Check sheet for the drawn part. Datum: minimum x, y, z corner. Units: mm. A direction names the side the tool comes from. Give positions to 0.01 mm unless a question says otherwise; leave off trailing zeros. Write each loop counter-clockwise with the first axis right and the second up, starting at its lowest first coordinate (ties: lowest second). Pieces come first, ordered by that corner, then holes. Notation, with made-up numbers: M 82,28.5 L 116,28.5 A18 ccw 116,34.5 Z; hole C -40,-39 d3. An arc over 180 degrees is marked long. Use CSV: the item, a comma, the result in double quotes. Start each with the question number.
1. Access from +Z, -Z, +X, -X, +Y, -Y to the whole of each face (thin tool, end or side, straight path). Record for the marked faces 1, 2 and 3.
2. Cross-section at B-B, the plane z = 13.7. Enter the section's corners in (x, y).
3. Depth check by flat-ended pin: P1, Ø5, axis at x = 3.5, z = 14, coming from the -Y side; P2, Ø12, axis at x = 6.5, y = 39, coming from the +Z side; P3, Ø12, axis at y = 25.5, z = 5, coming from the -X side. Enter the tip coordinate at first touch or a pass-through.
4. Cross-section at C-C, the plane y = 18. Enter the section's corners in (x, z), and give its area (3 significant figures).
5. Cross-section at A-A, the plane x = 13.7. Enter the section's corners in (y, z).
6. Cross-section at D-D, the plane y = 43.5. Enter the section's corners in (x, z).
7. Scan lines: line 1 (Y direction, x = 13, z = 20.75); line 2 (Y direction, x = 17.5, z = 12); line 3 (X direction, y = 6.5, z = 14.75). Record each from-to range of solid material in increasing order.
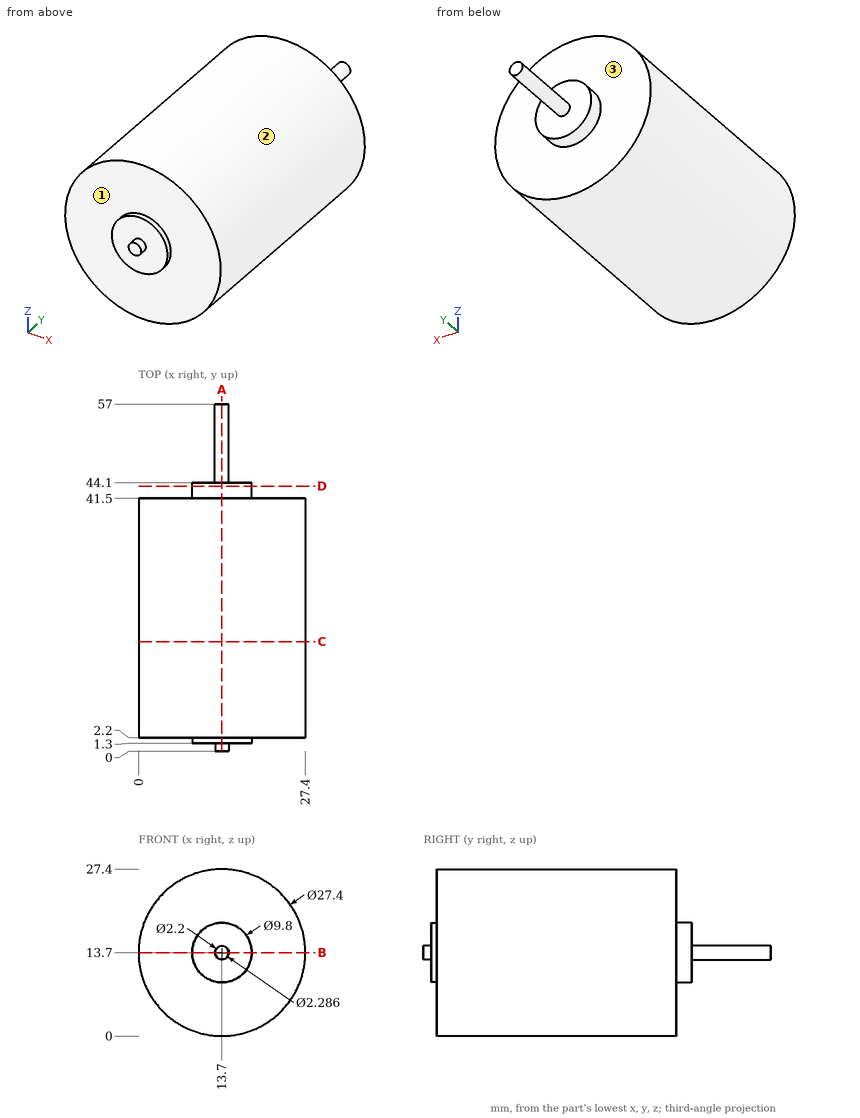
Worked answers:
1,face 1,"-Y"
1,face 2,"+Y, -Y"
1,face 3,"+Y"
2,outline,"M 0,2.2 L 8.8,2.2 L 8.8,1.3 L 12.6,1.3 L 12.6,0 L 14.8,0 L 14.8,1.3 L 18.6,1.3 L 18.6,2.2 L 27.4,2.2 L 27.4,41.5 L 18.6,41.5 L 18.6,44.1 L 14.84,44.1 L 14.84,57 L 12.56,57 L 12.56,44.1 L 8.8,44.1 L 8.8,41.5 L 0,41.5 Z"
3,P1,"stops at y = 2.2"
3,P2,"stops at z = 27.35"
3,P3,"stops at x = 0.27"
4,outline,"C 13.7,13.7 d27.4"
4,area,"590 mm^2"
5,outline,"M 0,12.6 L 1.3,12.6 L 1.3,8.8 L 2.2,8.8 L 2.2,0 L 41.5,0 L 41.5,8.8 L 44.1,8.8 L 44.1,12.56 L 57,12.56 L 57,14.84 L 44.1,14.84 L 44.1,18.6 L 41.5,18.6 L 41.5,27.4 L 2.2,27.4 L 2.2,18.6 L 1.3,18.6 L 1.3,14.8 L 0,14.8 Z"
6,outline,"C 13.7,13.7 d9.8"
7,line 1,"y = 2.2 to 41.5"
7,line 2,"y = 1.3 to 44.1"
7,line 3,"x = 0.04 to 27.36"
